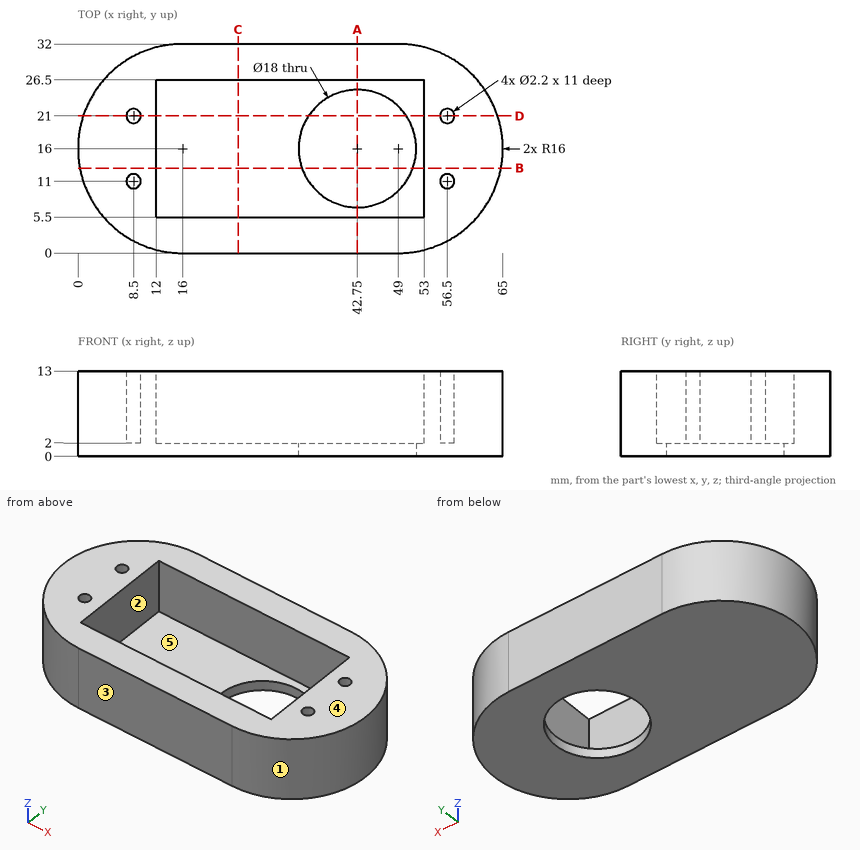
For this review, use the dimensioned drawing (mm, ordinates from the lowest corner) and the shaded views. A direction names the side the tool comes from. Coordinates: 2 decimals unless noted, no trailing zeros. Loops run counter-clockwise (first coordinate to the right, second up) from the corner with the lowest first, then second, coordinate; pieces in that order, holes last. Notation, with made-up numbers: (11.25, 72.5) - (52.25, 72.5) arc R33 cw to (52.25, 106.5) - close; hole circle Ø11 at (-17.5, -11.5). An arc over 180 degrees is marked (long way). Use CSV: the item, a comma, the result in double quotes. Start each with the question number.
1) Consider section B-B on y = 13. Write out the cut boundary in (x, z), then the cut area to 3 significant figures.
2) Consider section D-D on y = 21. Write out the cut boundary in (x, z), then the cut area to 3 significant figures.
3) The part is to be moulded in two halves that separate along X. For the marked faces 1, 2 and 3, say which applies: +X half, -X half, draft (parallel to the pull), parting line (faces both ways), or undercut.
4) Wall thickness on L1, parallel to Y at x = 42.5, z = 8.5; L2, parallel to X at y = 16, z = 6.5; L3, parallel to Y at x = 42.75, z = 0.7: over which ranges is each line inside the solid? List them lowest first. Write a range as from..to.
5) Consider section C-C on x = 24.5. Write out the cut boundary in (y, z).
6) Tool access review of the marked faces 4 and 5: name each direction out of +Z, -Z, +X, -X, +Y, -Y from which nothing blocks a thin tool from reaching the whole face with its end or side.
7) Consider section A-A on x = 42.75. Write out the cut boundary in (y, z).
8) For pin 1 Ø3 at (y, z) = (15.5, 7.5) entering from +X; pin 2 Ø0.7 at (x, y) = (57, 21.5) entering from +Z; pin 3 Ø6 at (x, z) = (11.5, 4) entering from -Y; pin 4 Ø1 at (y, z) = (22, 11) entering from +X (3 decimals), all flat-tipped, find the tip position at first contact; note any pin that passes through.
Geometry says:
1,outline,"(0.28, 0) - (34.26, 0) - (34.26, 2) - (12, 2) - (12, 13) - (0.28, 13) - close; (51.24, 0) - (64.72, 0) - (64.72, 13) - (53, 13) - (53, 2) - (51.24, 2) - close"
1,area,"353 mm^2"
2,outline,"(0.8, 0) - (35.27, 0) - (35.27, 2) - (12, 2) - (12, 13) - (9.6, 13) - (9.6, 2) - (7.4, 2) - (7.4, 13) - (0.8, 13) - close; (50.23, 0) - (64.2, 0) - (64.2, 13) - (57.6, 13) - (57.6, 2) - (55.4, 2) - (55.4, 13) - (53, 13) - (53, 2) - (50.23, 2) - close"
2,area,"295 mm^2"
3,face 1,"+X half"
3,face 2,"undercut"
3,face 3,"draft"
4,L1,"0..5.5, 26.5..32"
4,L2,"0..12, 53..65"
4,L3,"0..7, 25..32"
5,outline,"(0, 0) - (32, 0) - (32, 13) - (26.5, 13) - (26.5, 2) - (5.5, 2) - (5.5, 13) - (0, 13) - close"
6,face 4,"+Z, +X, -X, +Y, -Y"
6,face 5,"+Z"
7,outline,"(0, 0) - (7, 0) - (7, 2) - (5.5, 2) - (5.5, 13) - (0, 13) - close; (25, 0) - (32, 0) - (32, 13) - (26.5, 13) - (26.5, 2) - (25, 2) - close"
8,pin 1,"x = 65"
8,pin 2,"z = 2"
8,pin 3,"y = 0.07"
8,pin 4,"x = 64.025"
